from build123d import *

# Parameters (mm, degrees)
SKETCH1_R            = 2.5
BOSS_EXTRUDE1_DEPTH  = 2
CUT_EXTRUDE1_DEPTH   = 2
LPATTERN2_COUNT      = 4
LPATTERN2_PITCH      = 4
LPATTERN2_COL_COUNT  = 4
LPATTERN2_COL_PITCH  = 4
MIRROR2_COPY_1_DEPTH = 2
MIRROR2_COPY_2_DEPTH = 2
MIRROR2_COPY_3_DEPTH = 2
MIRROR2_COPY_4_DEPTH = 2
MIRROR2_COPY_5_DEPTH = 2
MIRROR2_COPY_6_DEPTH = 2
CUT_EXTRUDE3_DEPTH   = 2


with BuildPart() as part:
    # Sketch1 → Boss-Extrude1 (new body)
    with BuildSketch(Plane(origin=(0, 0, 0), x_dir=(1, 0, 0), z_dir=(0, 1, 0))):
        with BuildLine():
            Line((-6, -22.5), (6, -22.5))
            ThreePointArc((6, -22.5), (9.535533906, -21.035533906), (11, -17.5))
            Line((11, -17.5), (11, 17.5))
            ThreePointArc((11, 17.5), (9.535533906, 21.035533906), (6, 22.5))
            Line((6, 22.5), (-6, 22.5))
            ThreePointArc((-6, 22.5), (-9.535533906, 21.035533906), (-11, 17.5))
            Line((-11, 17.5), (-11, -17.5))
            ThreePointArc((-11, -17.5), (-9.535533906, -21.035533906), (-6, -22.5))
        make_face()
        with Locations(Location((0, 17.5, 0), (0, 0, 270))):
            Circle(SKETCH1_R, mode=Mode.SUBTRACT)
        with Locations(Location((0, -17.5, 0), (0, 0, 270))):
            Circle(SKETCH1_R, mode=Mode.SUBTRACT)
    extrude(amount=BOSS_EXTRUDE1_DEPTH)

    # Sketch2 → Cut-Extrude1 (cut)
    with BuildSketch(Plane(origin=(0, 2, 0), x_dir=(1, 0, 0), z_dir=(0, 1, 0))):
        with BuildLine():
            Line((-11, -1.85), (-11, 1.85))
            ThreePointArc((-11, 1.85), (-10.765685425, 1.284314575), (-10.2, 1.05))
            Line((-10.2, 1.05), (-9.3, 1.05))
            ThreePointArc((-9.3, 1.05), (-8.734314575, 0.815685425), (-8.5, 0.25))
            Line((-8.5, 0.25), (-8.5, -0.25))
            ThreePointArc((-8.5, -0.25), (-8.734314575, -0.815685425), (-9.3, -1.05))
            Line((-9.3, -1.05), (-10.2, -1.05))
            ThreePointArc((-10.2, -1.05), (-10.765685425, -1.284314575), (-11, -1.85))
        make_face()
    cut_extrude1 = extrude(amount=-CUT_EXTRUDE1_DEPTH, mode=Mode.SUBTRACT)

    # LPattern2: Cut-Extrude1 ×4
    with Locations(*[(0, 0, i * LPATTERN2_PITCH) for i in range(1, LPATTERN2_COUNT)]):
        add(cut_extrude1, mode=Mode.SUBTRACT)

    # LPattern2 col: Cut-Extrude1 ×4
    with Locations(*[(0, 0, -i * LPATTERN2_COL_PITCH) for i in range(1, LPATTERN2_COL_COUNT)]):
        add(cut_extrude1, mode=Mode.SUBTRACT)

    # Mirror2: Cut-Extrude1 across plane
    add(cut_extrude1.mirror(Plane(origin=(0, 0, 0), x_dir=(0, 0, 1), z_dir=(1, 0, 0))), mode=Mode.SUBTRACT)

    # Mirror2 copy 1 sketch → Mirror2 copy 1 (cut)
    with BuildSketch(Plane(origin=(0, 2, 4), x_dir=(-1, 0, 0), z_dir=(0, 1, 0))):
        with BuildLine():
            Line((-11, 1.85), (-11, -1.85))
            ThreePointArc((-11, -1.85), (-10.765685425, -1.284314575), (-10.2, -1.05))
            Line((-10.2, -1.05), (-9.3, -1.05))
            ThreePointArc((-9.3, -1.05), (-8.734314575, -0.815685425), (-8.5, -0.25))
            Line((-8.5, -0.25), (-8.5, 0.25))
            ThreePointArc((-8.5, 0.25), (-8.734314575, 0.815685425), (-9.3, 1.05))
            Line((-9.3, 1.05), (-10.2, 1.05))
            ThreePointArc((-10.2, 1.05), (-10.765685425, 1.284314575), (-11, 1.85))
        make_face()
    extrude(amount=-MIRROR2_COPY_1_DEPTH, mode=Mode.SUBTRACT)

    # Mirror2 copy 2 sketch → Mirror2 copy 2 (cut)
    with BuildSketch(Plane(origin=(0, 2, 8), x_dir=(-1, 0, 0), z_dir=(0, 1, 0))):
        with BuildLine():
            Line((-11, 1.85), (-11, -1.85))
            ThreePointArc((-11, -1.85), (-10.765685425, -1.284314575), (-10.2, -1.05))
            Line((-10.2, -1.05), (-9.3, -1.05))
            ThreePointArc((-9.3, -1.05), (-8.734314575, -0.815685425), (-8.5, -0.25))
            Line((-8.5, -0.25), (-8.5, 0.25))
            ThreePointArc((-8.5, 0.25), (-8.734314575, 0.815685425), (-9.3, 1.05))
            Line((-9.3, 1.05), (-10.2, 1.05))
            ThreePointArc((-10.2, 1.05), (-10.765685425, 1.284314575), (-11, 1.85))
        make_face()
    extrude(amount=-MIRROR2_COPY_2_DEPTH, mode=Mode.SUBTRACT)

    # Mirror2 copy 3 sketch → Mirror2 copy 3 (cut)
    with BuildSketch(Plane(origin=(0, 2, 12), x_dir=(-1, 0, 0), z_dir=(0, 1, 0))):
        with BuildLine():
            Line((-11, 1.85), (-11, -1.85))
            ThreePointArc((-11, -1.85), (-10.765685425, -1.284314575), (-10.2, -1.05))
            Line((-10.2, -1.05), (-9.3, -1.05))
            ThreePointArc((-9.3, -1.05), (-8.734314575, -0.815685425), (-8.5, -0.25))
            Line((-8.5, -0.25), (-8.5, 0.25))
            ThreePointArc((-8.5, 0.25), (-8.734314575, 0.815685425), (-9.3, 1.05))
            Line((-9.3, 1.05), (-10.2, 1.05))
            ThreePointArc((-10.2, 1.05), (-10.765685425, 1.284314575), (-11, 1.85))
        make_face()
    extrude(amount=-MIRROR2_COPY_3_DEPTH, mode=Mode.SUBTRACT)

    # Mirror2 copy 4 sketch → Mirror2 copy 4 (cut)
    with BuildSketch(Plane(origin=(0, 2, -4), x_dir=(-1, 0, 0), z_dir=(0, 1, 0))):
        with BuildLine():
            Line((-11, 1.85), (-11, -1.85))
            ThreePointArc((-11, -1.85), (-10.765685425, -1.284314575), (-10.2, -1.05))
            Line((-10.2, -1.05), (-9.3, -1.05))
            ThreePointArc((-9.3, -1.05), (-8.734314575, -0.815685425), (-8.5, -0.25))
            Line((-8.5, -0.25), (-8.5, 0.25))
            ThreePointArc((-8.5, 0.25), (-8.734314575, 0.815685425), (-9.3, 1.05))
            Line((-9.3, 1.05), (-10.2, 1.05))
            ThreePointArc((-10.2, 1.05), (-10.765685425, 1.284314575), (-11, 1.85))
        make_face()
    extrude(amount=-MIRROR2_COPY_4_DEPTH, mode=Mode.SUBTRACT)

    # Mirror2 copy 5 sketch → Mirror2 copy 5 (cut)
    with BuildSketch(Plane(origin=(0, 2, -8), x_dir=(-1, 0, 0), z_dir=(0, 1, 0))):
        with BuildLine():
            Line((-11, 1.85), (-11, -1.85))
            ThreePointArc((-11, -1.85), (-10.765685425, -1.284314575), (-10.2, -1.05))
            Line((-10.2, -1.05), (-9.3, -1.05))
            ThreePointArc((-9.3, -1.05), (-8.734314575, -0.815685425), (-8.5, -0.25))
            Line((-8.5, -0.25), (-8.5, 0.25))
            ThreePointArc((-8.5, 0.25), (-8.734314575, 0.815685425), (-9.3, 1.05))
            Line((-9.3, 1.05), (-10.2, 1.05))
            ThreePointArc((-10.2, 1.05), (-10.765685425, 1.284314575), (-11, 1.85))
        make_face()
    extrude(amount=-MIRROR2_COPY_5_DEPTH, mode=Mode.SUBTRACT)

    # Mirror2 copy 6 sketch → Mirror2 copy 6 (cut)
    with BuildSketch(Plane(origin=(0, 2, -12), x_dir=(-1, 0, 0), z_dir=(0, 1, 0))):
        with BuildLine():
            Line((-11, 1.85), (-11, -1.85))
            ThreePointArc((-11, -1.85), (-10.765685425, -1.284314575), (-10.2, -1.05))
            Line((-10.2, -1.05), (-9.3, -1.05))
            ThreePointArc((-9.3, -1.05), (-8.734314575, -0.815685425), (-8.5, -0.25))
            Line((-8.5, -0.25), (-8.5, 0.25))
            ThreePointArc((-8.5, 0.25), (-8.734314575, 0.815685425), (-9.3, 1.05))
            Line((-9.3, 1.05), (-10.2, 1.05))
            ThreePointArc((-10.2, 1.05), (-10.765685425, 1.284314575), (-11, 1.85))
        make_face()
    extrude(amount=-MIRROR2_COPY_6_DEPTH, mode=Mode.SUBTRACT)

    # Sketch4 → Cut-Extrude3 (cut)
    with BuildSketch(Plane(origin=(0, 2, 0), x_dir=(1, 0, 0), z_dir=(0, 1, 0))):
        with BuildLine():
            Line((-1.5, -10), (1.5, -10))
            ThreePointArc((1.5, -10), (5.035533906, -8.535533906), (6.5, -5))
            Line((6.5, -5), (6.5, 5))
            ThreePointArc((6.5, 5), (5.035533906, 8.535533906), (1.5, 10))
            Line((1.5, 10), (-1.5, 10))
            ThreePointArc((-1.5, 10), (-5.035533906, 8.535533906), (-6.5, 5))
            Line((-6.5, 5), (-6.5, -5))
            ThreePointArc((-6.5, -5), (-5.035533906, -8.535533906), (-1.5, -10))
        make_face()
    extrude(amount=-CUT_EXTRUDE3_DEPTH, mode=Mode.SUBTRACT)


solid = part.part
Could you check a few things on this model? Use its own coordinates, in mm. A direction names the side the tool comes from. Round coordinates to 2 decimals unless told otherwise and drop trailing zeros. Order: outer loops, then holes, each group sorted by start corner. A loop starts at its lowest first (then second) coordinate and runs counter-clockwise, first axis right, second up. Notation, with made-up numbers: M 12,31.25 L 27,31.25 A25 cw 27,43.25 Z; hole C -25.5,51.25 d7. An arc over 180 degrees is marked long. One line per item, written item: value.
(1) Imagine slicing it at C-C (y = 0.35). Count the separate pieces of the cut face and the enclosed holes in it, and give its area (3 significant figures).
Ans:
separate pieces: 1
enclosed holes: 3
area: 617 mm^2
(2) I'm going to push flat-ended pins straight in: P1, Ø0.7, axis at x = 10, y = 1.5, coming from the -Z side; P2, Ø1, axis at x = -9.5, y = 0.5, coming from the -Z side; P3, Ø1, axis at x = 10, y = 1, coming from the +Z side. Where does each tip first touch, or does it pass through?
Ans:
P1: stops at z = -20.92
P2: stops at z = -21.5
P3: stops at z = 21.07
(3) Imagine slicing it at B-B (x = 0). Write out the boundary of the cut face in (y, z), and give its area (3 significant figures).
Ans:
outline: M 0,-22.5 L 2,-22.5 L 2,-20 L 0,-20 Z; M 0,-15 L 2,-15 L 2,-10 L 0,-10 Z; M 0,10 L 2,10 L 2,15 L 0,15 Z; M 0,20 L 2,20 L 2,22.5 L 0,22.5 Z
area: 30.0 mm^2
(4) Imagine slicing it at D-D (x = -3.5). Write out the boundary of the cut face in (y, z).
Ans:
outline: M 0,-22.5 L 2,-22.5 L 2,-9.58 L 0,-9.58 Z; M 0,9.58 L 2,9.58 L 2,22.5 L 0,22.5 Z
(5) Which directions (+Z, -Z, +X, -X, +Y, -Y) give clear straight access to the entire face, cutting with the end or side of a thin tool? Please do faces 4 (the cylindrical face through (-8.73, 1.01, 4.81)), 5 (the flat face through (10, 1, -6.95)), 6 (the flat face through (-7, 0, 0)).
Ans:
face 4: -X, +Y, -Y
face 5: +X, +Y, -Y
face 6: +Z, -Z, +X, -X, -Y
(6) Imagine slicing it at A-A (x = 4.5). Write out the boundary of the cut face in (y, z).
Ans:
outline: M 0,-22.5 L 2,-22.5 L 2,-9 L 0,-9 Z; M 0,9 L 2,9 L 2,22.5 L 0,22.5 Z
(7) I need wall thicknesses on line 1 along X through (y, z) = (0.9, -17.5); line 2 along X through (y, z) = (0.9, -2); line 3 along X through (y, z) = (0.7, -13.5). Which ranges of each line are inside material? Lowest first, please. Write a range as from..to.
Ans:
line 1: x = -11..-2.5, 2.5..11
line 2: x = -11..-6.5, 6.5..11
line 3: x = -10.92..10.92
(8) If we mould it in two halves opening along X, with no side actions, what happens to faces 1 (the cylindrical face through (8.74, 1.01, -8.82)), 2 (the cylindrical face through (-10.76, 1.01, -2.72)), 3 (the flat face through (-6.5, 1, 0))? For each: released by +X, released by -X, zero draft, split by the parting line, or undercut.
Ans:
face 1: released by +X
face 2: released by -X
face 3: undercut
